The drawing under review shows one solid part. Ordinate dimensions are in mm from its lowest x, y, z. A direction names the side the tool comes from. Round coordinates to 2 decimals unless told otherwise and drop trailing zeros. Order: outer loops, then holes, each group sorted by start corner. A loop starts at its lowest first (then second) coordinate and runs counter-clockwise, first axis right, second up. Notation, with made-up numbers: M -20.5,-40 L 14.5,-40 A15 ccw 14.5,-15 Z; hole C 28.5,-11.75 d9. An arc over 180 degrees is marked long. Answer in a Markdown table with one row per item. Add a question column.
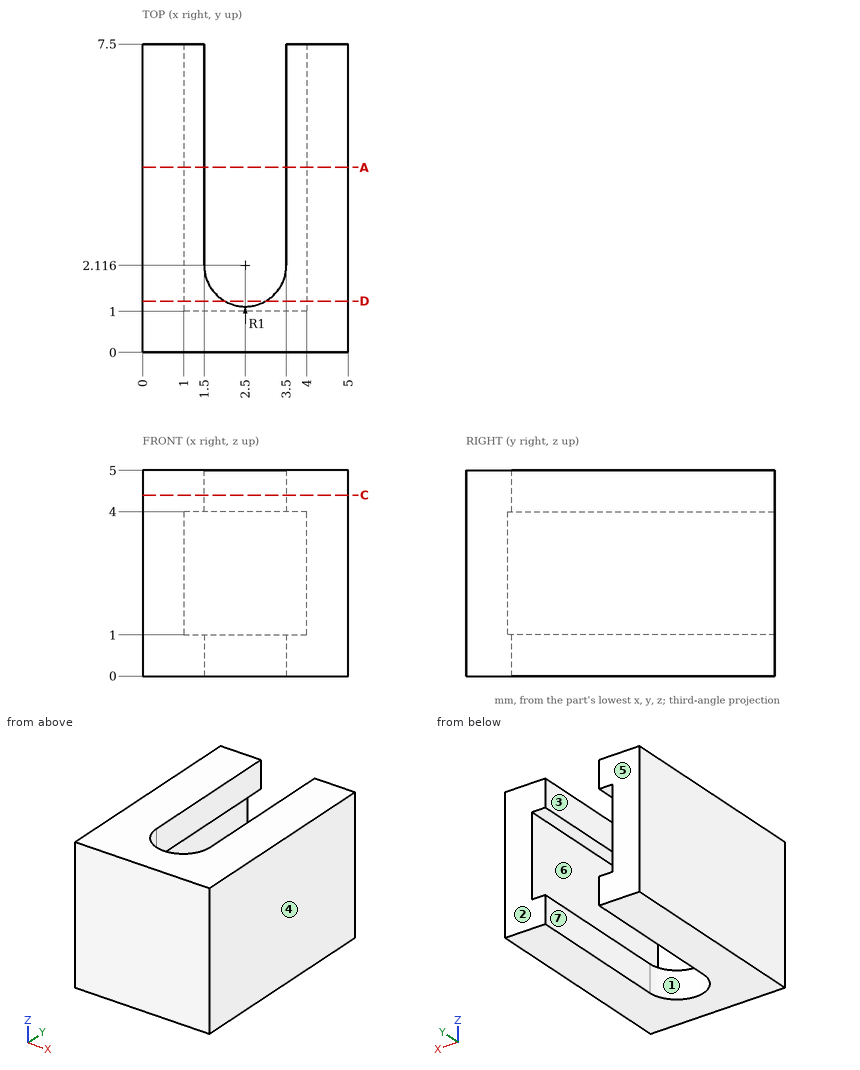
1. Consider section D-D on y = 1.25. Write out the cut boundary in (x, z), plus the area to 3 significant figures.
2. Consider section C-C on z = 4.4. Write out the cut boundary in (x, y) (1 decimal).
3. The part is to be moulded in two halves that separate along X. For the marked faces 1, 2, 3 and 4, say which applies: pulls with the +X half, pulls with the -X half, needs draft (parallel to the pull), parting line crosses it, or undercut.
4. For the marked faces 5, 6 and 7, list the 3-axis set-ups (+Z, -Z, +X, -X, +Y, -Y) from which the entire face can be reached by the end or side of a thin tool; tool diameter is ignored.
5. Consider section A-A on y = 4.5. Write out the cut boundary in (x, z), plus the area to 3 significant figures.
6. To check wall thickness, follow probe 1 along Z at (x, y) = (1.35, 4.5); probe 2 along X at (y, z) = (7, 4.25). State the ranges of each line that lie inside material, in increasing order. Write a range as [from, to].
Solved:
| question | item | result |
|---|---|---|
| 1 | outline | M 0,0 L 2,0 L 2,1 L 1,1 L 1,4 L 2,4 L 2,5 L 0,5 Z; M 3,0 L 5,0 L 5,5 L 3,5 L 3,4 L 4,4 L 4,1 L 3,1 Z |
| 1 | area | 14.0 mm^2 |
| 2 | outline | M 0,0 L 5,0 L 5,7.5 L 3.5,7.5 L 3.5,2.1 A1 cw 1.5,2.1 L 1.5,7.5 L 0,7.5 Z |
| 3 | face 1 | undercut |
| 3 | face 2 | needs draft |
| 3 | face 3 | undercut |
| 3 | face 4 | pulls with the +X half |
| 4 | face 5 | +Z, -Z, +X, -X, +Y |
| 4 | face 6 | +Y |
| 4 | face 7 | +Z, -Z, +Y |
| 5 | outline | M 0,0 L 1.5,0 L 1.5,1 L 1,1 L 1,4 L 1.5,4 L 1.5,5 L 0,5 Z; M 3.5,0 L 5,0 L 5,5 L 3.5,5 L 3.5,4 L 4,4 L 4,1 L 3.5,1 Z |
| 5 | area | 12.0 mm^2 |
| 6 | probe 1 | z = [0, 1], [4, 5] |
| 6 | probe 2 | x = [0, 1.5], [3.5, 5] |
